Can you work these out from the drawing? Everything is in mm from the part's minimum corner. Give positions to 0.01 mm unless a question says otherwise; leave off trailing zeros. Loops run counter-clockwise (first coordinate to the right, second up) from the corner with the lowest first, then second, coordinate; pieces in that order, holes last. Notation, with made-up numbers: (-31.75, 82) -> (12.25, 82) arc R33 cw to (12.25, 121) -> close; hole circle Ø10 at (80, 18.25). An arc over 180 degrees is marked (long way). Write item = value, one per line. Start each with the question number.
1) I want a section at B-B (x = 20). List the corners of the cut face in (y, z) for me.
2) I need wall thicknesses on probe 1 along Y at (x, z) = (2, 1.2); probe 2 along Y at (x, z) = (19.5, 1.2). Which ranges of each line are inside material? Lowest first, please. Write a range as from..to.
3) I want a section at C-C (z = 0.45). List the corners of the cut face in (x, y) for me, and give its area (3 significant figures).
4) I want a section at A-A (y = 15). List the corners of the cut face in (x, z) for me.
5) I'm going to push a flat-ended pin straight in: pin 1 Ø1.9 at (x, y) = (20, 15) entering from +Z. Where does the tip first touch, or does it pass through?
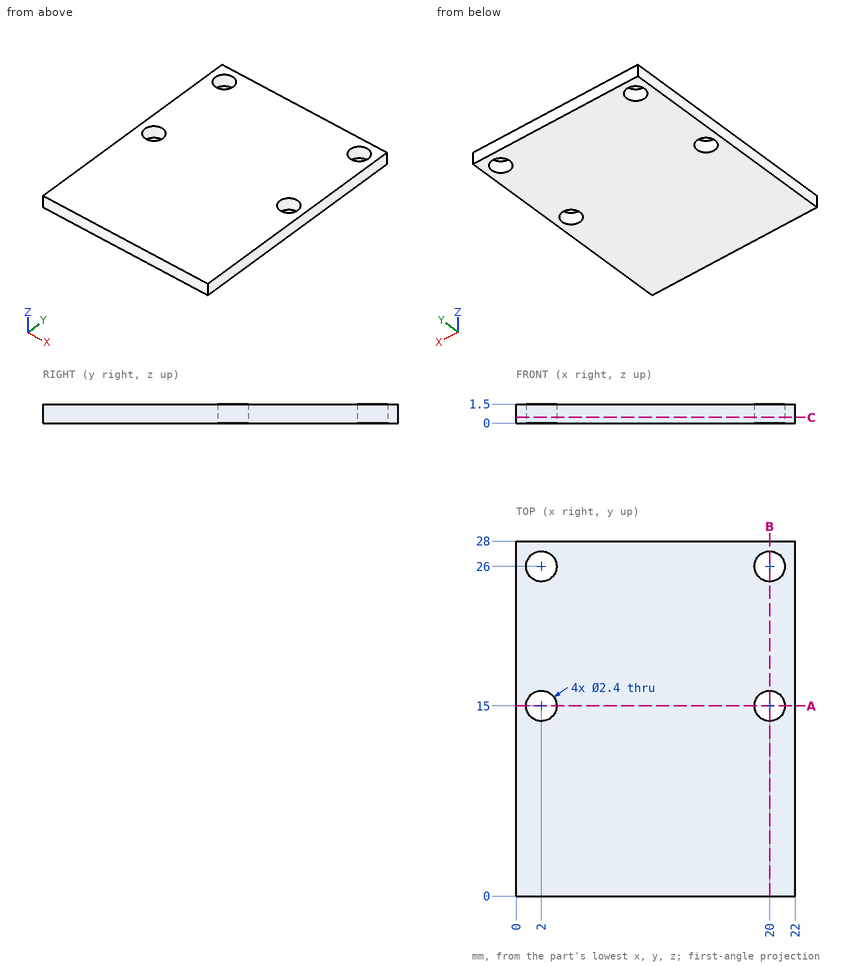
Answer list:
q1.outline = (0, 0) -> (13.8, 0) -> (13.8, 1.5) -> (0, 1.5) -> close; (16.2, 0) -> (24.8, 0) -> (24.8, 1.5) -> (16.2, 1.5) -> close; (27.2, 0) -> (28, 0) -> (28, 1.5) -> (27.2, 1.5) -> close
q2.probe_1 = 0..13.8, 16.2..24.8, 27.2..28
q2.probe_2 = 0..13.91, 16.09..24.91, 27.09..28
q3.outline = (0, 0) -> (22, 0) -> (22, 28) -> (0, 28) -> close; hole circle Ø2.4 at (2, 15); hole circle Ø2.4 at (2, 26); hole circle Ø2.4 at (20, 15); hole circle Ø2.4 at (20, 26)
q3.area = 598 mm^2
q4.outline = (0, 0) -> (0.8, 0) -> (0.8, 1.5) -> (0, 1.5) -> close; (3.2, 0) -> (18.8, 0) -> (18.8, 1.5) -> (3.2, 1.5) -> close; (21.2, 0) -> (22, 0) -> (22, 1.5) -> (21.2, 1.5) -> close
q5.pin_1 = through
